Autodesk Inventor part; units mm, degrees
ref_plane "YZ Plane" through (0, 0, 0) normal (1, 0, 0) x (0, 1, 0)
ref_plane "XZ Plane" through (0, 0, 0) normal (0, 1, 0) x (-1, 0, 0)
ref_plane "XY Plane" through (0, 0, 0) normal (0, 0, 1) x (1, 0, 0)
sketch "スケッチ1" plane through (0, 0, 0) normal (0, 1, 0) x (-1, 0, 0)
  line L0 (-2, 7.5) -> (2, 7.5)
  line L1 (2, 7.5) -> (2, -7.5)
  line L2 (2, -7.5) -> (-2, -7.5)
  line L3 (-2, -7.5) -> (-2, 7.5)
  line L4 (-2, 7.5) -> (2, -7.5) construction
  line L5 (2, 7.5) -> (-2, -7.5) construction
  circle A0 centre (0, 5.5) radius 1
  circle A1 centre (0, -5.5) radius 1
  line L6 (0, 5.5) -> (0, 7.5) construction
  line L7 (0, -5.5) -> (0, -7.5) construction
  point P0 (0, 0)
  dimension "d0" = 4
  dimension "d1" = 15
  dimension "d2" = 2
  dimension "d3" = 2
extrude "押し出し1" add sketch "スケッチ1" along normal blind 30 contours L0 L1 L2 L3 | A0 | A1
extrude "押し出し2" cut sketch "スケッチ1" along normal blind 6 contours A0 | A1
sketch "スケッチ2" plane through (-2, 0, -7.5) normal (-1, 0, 0) x (0, 0, 1)
  line L0 (4, 12) -> (11, 12)
  line L1 (13, 14) -> (13, 22)
  line L2 (11, 24) -> (4, 24)
  line L3 (2, 22) -> (2, 14)
  arc A0 (2, 14) -> (4, 12) centre (4, 14) ccw
  arc A1 (4, 24) -> (2, 22) centre (4, 22) ccw
  arc A2 (13, 22) -> (11, 24) centre (11, 22) ccw
  arc A3 (11, 12) -> (13, 14) centre (11, 14) ccw
  line L4 (7.5, 0) -> (7.5, 30) construction
  line L5 (0, 30) -> (15, 30)
  circle A4 centre (4, 14) radius 0.8
  circle A5 centre (4, 22) radius 0.8
  circle A6 centre (11, 22) radius 0.8
  circle A7 centre (11, 14) radius 0.8
  point P0 (2, 12)
  point P1 (13, 24)
  point P2 (2, 24)
  dimension "d8" = 12
  dimension "d9" = 11
  dimension "d10" = 2
  dimension "d11" = 6
  dimension "d12" = 1.6
extrude "押し出し3" cut sketch "スケッチ2" against normal blind 1
extrude "押し出し4" cut sketch "スケッチ2" against normal up to surface (4 mm away) contours A4 | A5 | A6 | A7
properties part number "BallSensor_Mount"
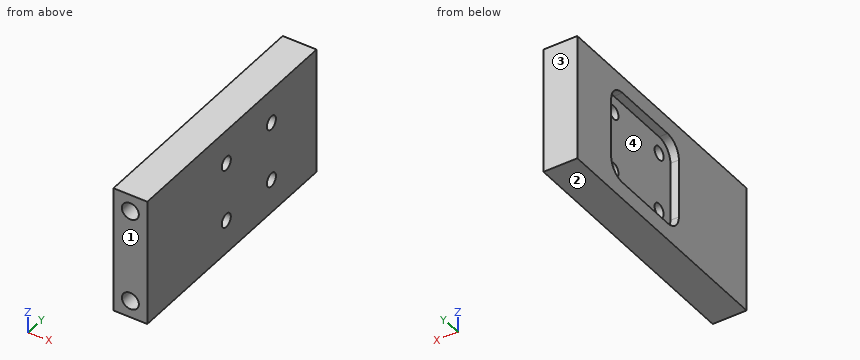
Build history of the part. All positions in model axes, mm. Face numbers are marked on the shaded views. Round coordinates to 2 decimals unless told otherwise and drop trailing zeros. Loops run counter-clockwise (first coordinate to the right, second up) from the corner with the lowest first, then second, coordinate; pieces in that order, holes last. Notation, with made-up numbers: (77.25, 53.25) -> (129.25, 53.25) arc R18 ccw to (129.25, 81.25) -> close; hole circle Ø10 at (34, -10.5). An arc over 180 degrees is marked (long way). Answer in a Markdown table with one row per item.
Item 1: Pin check, flat tips, straight feed: pin 1 (1 mm diameter, centred on y = 14, z = 3.5, fed in from +X); pin 2 (1.8 mm diameter, centred on y = 22, z = 3.5, fed in from -X). Stop position of each tip, or through.
Answers below:
| item | result |
|---|---|
| pin 1 | passes through |
| pin 2 | stops at x = -1 |
Item 2: Drill centre lines: L1, parallel to Y at x = 1.1, z = 3.5; L2, parallel to Z at x = 0, y = 3.3; L3, parallel to Y at x = -0.5, z = -4. Where is each one in solid material? Low to high. Write a range as [from, to].
Answers below:
| item | result |
|---|---|
| L1 | y = [0, 13.2], [14.8, 21.2], [22.8, 30] |
| L2 | z = [-7.5, -6.5], [-4.5, 4.5], [6.5, 7.5] |
| L3 | y = [0, 13.38], [14.62, 21.38], [22.62, 30] |
Item 3: Saw through at B-B (z = 2). Write the cut outline in (x, y), and give its area (3 significant figures).
Answers below:
| item | result |
|---|---|
| outline | (-2, 0) -> (2, 0) -> (2, 30) -> (-2, 30) -> (-2, 24) -> (-1, 24) -> (-1, 12) -> (-2, 12) -> close |
| area | 108 mm² |
Item 4: Saw through at C-C (y = 2.75). Write the cut outline in (x, z), and give its area (3 significant figures).
Answers below:
| item | result |
|---|---|
| outline | (-2, -7.5) -> (2, -7.5) -> (2, 7.5) -> (-2, 7.5) -> close; hole circle Ø2 at (0, -5.5); hole circle Ø2 at (0, 5.5) |
| area | 53.7 mm² |
Item 5: Mould opens along Y. For the marked faces 1, 2, 3 and 4 say: +Y half, -Y half, draft (parallel to the pull), parting line (faces both ways), or undercut.
Answers below:
| item | result |
|---|---|
| face 1 | -Y half |
| face 2 | draft |
| face 3 | +Y half |
| face 4 | undercut |
Item 6: Saw through at A-A (x = 0). Write the cut outline in (y, z).
Answers below:
| item | result |
|---|---|
| outline | (0, -7.5) -> (30, -7.5) -> (30, 7.5) -> (0, 7.5) -> (0, 6.5) -> (6, 6.5) -> (6, 4.5) -> (0, 4.5) -> (0, -4.5) -> (6, -4.5) -> (6, -6.5) -> (0, -6.5) -> close; hole circle Ø1.6 at (14, -3.5); hole circle Ø1.6 at (14, 3.5); hole circle Ø1.6 at (22, -3.5); hole circle Ø1.6 at (22, 3.5) |
Item 7: Saw through at D-D (x = -1.5). Write the cut outline in (y, z), and give its area (3 significant figures).
Answers below:
| item | result |
|---|---|
| outline | (0, -7.5) -> (30, -7.5) -> (30, 7.5) -> (0, 7.5) -> close; hole (12, -3.5) arc R2 ccw to (14, -5.5) -> (22, -5.5) arc R2 ccw to (24, -3.5) -> (24, 3.5) arc R2 ccw to (22, 5.5) -> (14, 5.5) arc R2 ccw to (12, 3.5) -> close |
| area | 321 mm² |
